The drawing under review shows one solid part. Ordinate dimensions are in mm from its lowest x, y, z. Round coordinates to 2 decimals unless told otherwise and drop trailing zeros. Order: outer loops, then holes, each group sorted by start corner. A loop starts at its lowest first (then second) coordinate and runs counter-clockwise, first axis right, second up. Notation, with made-up numbers: (-11.75, 83) - (31.25, 83) arc R30 ccw to (31.25, 114) - close; hole circle Ø9 at (-36.5, 53). An arc over 180 degrees is marked (long way). One line per question, with ' | ' between items.
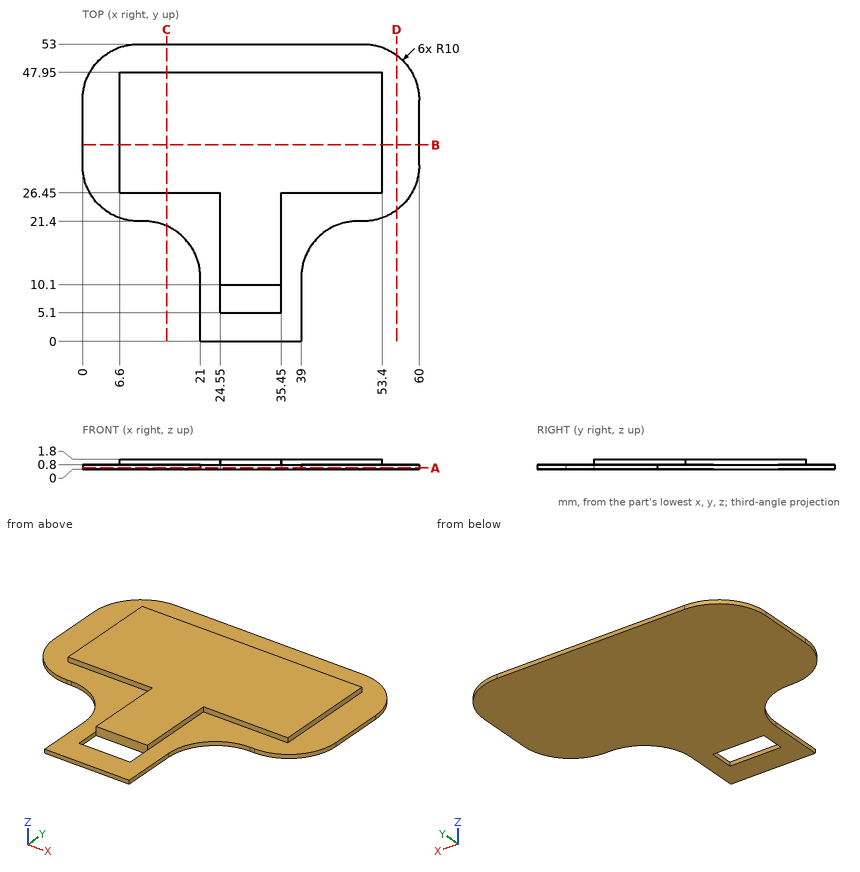
(1) We need section C-C on x = 15. State the section outline as (y, z) points, plus the area to 3 significant figures.
Output values:
outline: (20.57, 0) - (53, 0) - (53, 0.8) - (47.95, 0.8) - (47.95, 1.8) - (26.45, 1.8) - (26.45, 0.8) - (20.57, 0.8) - close | area: 47.4 mm^2
(2) We need section D-D on x = 56. State the section outline as (y, z) points.
Output values:
outline: (23.4, 0) - (51, 0) - (51, 0.8) - (23.4, 0.8) - close
(3) We need section B-B on y = 35. State the section outline as (x, z) points.
Output values:
outline: (0, 0) - (60, 0) - (60, 0.8) - (53.4, 0.8) - (53.4, 1.8) - (6.6, 1.8) - (6.6, 0.8) - (0, 0.8) - close
(4) Insertion check: pin 1 (2 mm diameter, centred on x = 10, y = 24.5, fed in from +Z); pin 2 (1 mm diameter, centred on x = 44.5, y = 38, fed in from -Z); pin 3 (0.9 mm diameter, centred on y = 8, z = 0.5, fed in from +X). Each pin has a flat end and moves straight along its axis. Give the tip position at first contact, or say it passes through.
Output values:
pin 1: z = 0.8 | pin 2: z = 0 | pin 3: x = 39
(5) For probe 1 along Y at (x, z) = (30, 0.65); probe 2 along Y at (x, z) = (18, 1.6); probe 3 along X at (y, z) = (17, 1.6), list the stretches that pass through material, from the lowest coordinate up. Write a range as [from, to].
Output values:
probe 1: [0, 5.1], [10.1, 53] | probe 2: [26.45, 47.95] | probe 3: [24.55, 35.45]
(6) We need section A-A on z = 0.3. State the section outline as (x, y) points.
Output values:
outline: (0, 31.4) arc R10 ccw to (10, 21.4) - (11, 21.4) arc R10 cw to (21, 11.4) - (21, 0) - (39, 0) - (39, 11.4) arc R10 cw to (49, 21.4) - (50, 21.4) arc R10 ccw to (60, 31.4) - (60, 43) arc R10 ccw to (50, 53) - (10, 53) arc R10 ccw to (0, 43) - close; hole (24.55, 5.1) - (35.45, 5.1) - (35.45, 10.1) - (24.55, 10.1) - close
